Work out the finished part from the listing and answer in its coordinate system (mm). A direction names the side the tool comes from. Round coordinates to 2 decimals unless told otherwise and drop trailing zeros. Order: outer loops, then holes, each group sorted by start corner. A loop starts at its lowest first (then second) coordinate and runs counter-clockwise, first axis right, second up. Notation, with made-up numbers: (55, 75.5) - (95, 75.5) arc R35 ccw to (95, 111.5) - close; hole circle Ø9 at (-13, 47). An arc over 180 degrees is marked (long way). Use one line per item in the form item = value. Start each with the question number.
Q1. The part is cut by section A-A on y = 466. Determine the outline of the cut face in (x, z).
Q2. For a pull along Z with two mould halves and no side action, classify faces 1 (the flat face through (597, 0, 213)), 2 (the flat face through (608, 775, 750)), 3 (the flat face through (30, 615, 373)) as +Z half, -Z half, draft (parallel to the pull), parting line (faces both ways), or undercut.
Q3. Given P1, Ø2, axis at x = 589, y = 375.5, coming from the -Z side; P2, Ø12, axis at x = 835.5, y = 713.5, coming from the +Z side; P3, Ø25, axis at x = 1178.5, y = 500.5, coming from the +Z side, each flat-ended and moving along its own axis, determine where each tip first touches the part or whether it passes through.
Q4. The part is cut by section C-C on z = 475.5. State how many separate pieces and enclosed holes the cut face has, plus the area to 3 significant figures.
Q5. Find the intervals of material crossed by line 1 (X direction, y = 101.5, z = 331.5); line 2 (Y direction, x = 814.5, z = 359.5); line 3 (Z direction, x = 478.5, y = 765), in increasing order. Write a range as [from, to].
Q6. The part is cut by section B-B on x = 1062.5. Determine the outline of the cut face in (y, z), plus the area to 3 significant figures.
Q7. Which of the six approach directions +Z, -Z, +X, -X, +Y, -Y give full straight-line access (tool end or side, diameter ignored) to faces 4 (the flat face through (1185, 700, 373)), 5 (the flat face through (1170, 115, 373)), 6 (the flat face through (1030, 785, 472))?
from build123d import *

# Parameters (mm, degrees)
EXTRUDE_DEPTH    = 50
SKETCH001_W      = 1200
SKETCH001_H      = 800
EXTRUDE001_DEPTH = 30
EXTRUDE002_DEPTH = 50
SKETCH003_W      = 30
SKETCH003_H      = 30
EXTRUDE003_DEPTH = 290
ARRAY_Y_COUNT    = 8
ARRAY_Y_PITCH    = 100
EXTRUDE004_DEPTH = 490
ARRAY001_X_COUNT = 12
ARRAY001_X_PITCH = 100


with BuildPart() as extrude_body:
    # Sketch → Extrude (new body)
    with BuildSketch(Plane.YZ):
        Polygon((0, 0), (30, 0), (30, 520), (770, 520), (770, 0), (800, 0), (800, 550), (0, 550), align=None)
    extrude(amount=EXTRUDE_DEPTH)


with BuildPart() as extrude004:
    # Sketch001 → Extrude001 (new body)
    with BuildSketch(Plane.XY):
        with Locations((600, 400)):
            Rectangle(SKETCH001_W, SKETCH001_H)
    extrude(amount=EXTRUDE001_DEPTH)


with BuildPart() as extrude004_1:
    # Extrude001 placement: moved
    add(extrude004.part.moved(Location((0, 0, 200))))


with BuildPart() as extrude002:
    # Sketch002 → Extrude002 (new body)
    with BuildSketch(Plane.XZ):
        Polygon((0, 0), (50, 0), (50, 720), (1150, 720), (1150, 0), (1200, 0), (1200, 750), (0, 750), align=None)
    extrude(amount=EXTRUDE002_DEPTH)


with BuildPart() as extrude002_1:
    # Extrude002 placement: moved
    add(extrude002.part.moved(Location((0, 800, 0))))


with BuildPart() as array:
    # Sketch003 → Extrude003 (new body)
    with BuildSketch(Plane.XY):
        with Locations((15, 15)):
            Rectangle(SKETCH003_W, SKETCH003_H)
    extrude(amount=EXTRUDE003_DEPTH)

    # Array Y: Array ×8


with BuildPart() as array_1:
    add(array.part)
    with Locations(*[(0, i * ARRAY_Y_PITCH, 0) for i in range(1, ARRAY_Y_COUNT)]):
        add(array.part)


with BuildPart() as array_2:
    # Array placement: moved
    add(array_1.part.moved(Location((0, 0, 230))))


with BuildPart() as array001:
    # Clone001 base: copy of Array
    add(array_2.part)


with BuildPart() as array001_1:
    # Clone001 placement: moved
    add(array001.part.moved(Location((1170, 0, 0))))


with BuildPart() as array002:
    # Sketch003 → Extrude004 (new body)
    with BuildSketch(Plane.XY):
        with Locations((15, 15)):
            Rectangle(SKETCH003_W, SKETCH003_H)
    extrude(amount=EXTRUDE004_DEPTH)

    # Array001 X: Array002 ×12


with BuildPart() as array002_1:
    add(array002.part)
    with Locations(*[(i * ARRAY001_X_PITCH, 0, 0) for i in range(1, ARRAY001_X_COUNT)]):
        add(array002.part)


with BuildPart() as array002_2:
    # Array001 placement: moved
    add(array002_1.part.moved(Location((0, 770, 230))))


with BuildPart() as fusion:
    # Clone base: copy of Extrude body
    add(extrude_body.part)


with BuildPart() as fusion_1:
    # Clone placement: moved
    add(fusion.part.moved(Location((1150, 0, 0))))

    # Fusion: union Extrude body, Extrude004, Extrude002, Array, Array001, Array002
    add(extrude_body.part)
    add(extrude004_1.part)
    add(extrude002_1.part)
    add(array_2.part)
    add(array001_1.part)
    add(array002_2.part)


solid = fusion_1.part
Found:
q1.outline = (0, 200) - (1200, 200) - (1200, 230) - (0, 230) - close; (0, 520) - (50, 520) - (50, 550) - (0, 550) - close; (1150, 520) - (1200, 520) - (1200, 550) - (1150, 550) - close
q2.face_1 = draft
q2.face_2 = +Z half
q2.face_3 = undercut
q3.P1 = 200
q3.P2 = 230
q3.P3 = 550
q4.separate_pieces = 29
q4.enclosed_holes = 0
q4.area = 30,500 mm²
q5.line_1 = [0, 30], [1170, 1200]
q5.line_2 = [770, 800]
q5.line_3 = [200, 230], [720, 750]
q6.outline = (0, 200) - (800, 200) - (800, 230) - (0, 230) - close; (750, 720) - (800, 720) - (800, 750) - (750, 750) - close
q6.area = 25,500 mm²
q7.face_4 = +X, -X
q7.face_5 = none
q7.face_6 = +Y, -Y
